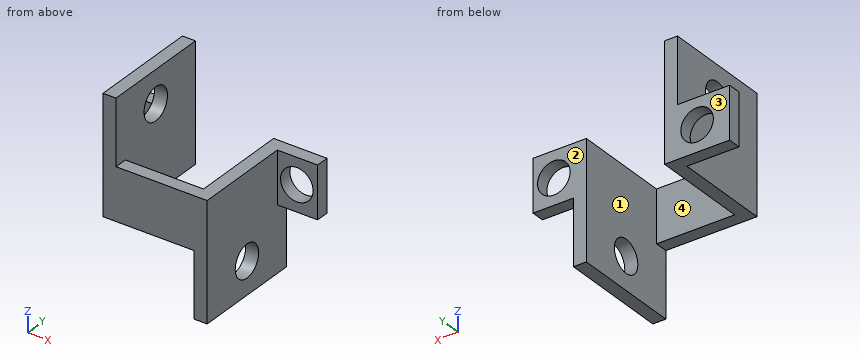
from build123d import *

# Parameters (mm, degrees)
CROQUIS1_W              = 8
CROQUIS1_H              = 2
SALIENTE_EXTRUIR1_DEPTH = 8
CROQUIS2_R              = 2.5
CORTAR_EXTRUIR1_DEPTH   = 2
SKETCH1_W               = 8
SKETCH1_H               = 2
CUT_EXTRUDE1_DEPTH      = 1.8
SKETCH5_W               = 10
SKETCH5_H               = 17
BOSS_EXTRUDE3_DEPTH     = 2
SKETCH6_W               = 10
SKETCH6_H               = 17
SKETCH6_R               = 2.5
BOSS_EXTRUDE4_DEPTH     = 2
SKETCH7_R               = 2.5
CUT_EXTRUDE2_DEPTH      = 2


with BuildPart() as part:
    # Croquis1 → Saliente-Extruir1 (new body)
    with BuildSketch(Plane.XY):
        with Locations((-12, 6.5)):
            Rectangle(CROQUIS1_W, CROQUIS1_H)
        Polygon((-6, 7.5), (-8, 7.5), (-8, 5.5), (-8, -9.5), (8, -9.5), (8, 5.5), (8, 7.5), (6, 7.5), (6, -7.5), (-6, -7.5), align=None)
        with Locations((12, 6.5)):
            Rectangle(CROQUIS1_W, CROQUIS1_H)
    extrude(amount=SALIENTE_EXTRUIR1_DEPTH)

    # Croquis2 → Cortar-Extruir1 (cut)
    with BuildSketch(Plane(origin=(0, 7.5, 0), x_dir=(1, 0, 0), z_dir=(0, 1, 0))):
        with Locations((-11, -4)):
            Circle(CROQUIS2_R)
        with Locations((11, -4)):
            Circle(CROQUIS2_R)
    extrude(amount=-CORTAR_EXTRUIR1_DEPTH, mode=Mode.SUBTRACT)

    # Sketch1 → Cut-Extrude1 (cut)
    with BuildSketch(Plane(origin=(16, 0, 0), x_dir=(0, 0, -1), z_dir=(1, 0, 0))):
        with Locations((-4, 6.5)):
            Rectangle(SKETCH1_W, SKETCH1_H)
    extrude(amount=-CUT_EXTRUDE1_DEPTH, mode=Mode.SUBTRACT)

    # Sketch5 → Boss-Extrude3 (add)
    with BuildSketch(Plane.ZY.offset(8)):
        with Locations((13, -1)):
            Rectangle(SKETCH5_W, SKETCH5_H)
    extrude(amount=-BOSS_EXTRUDE3_DEPTH)

    # Sketch6 → Boss-Extrude4 (add)
    with BuildSketch(Plane(origin=(8, 0, 0), x_dir=(0, 0, -1), z_dir=(1, 0, 0))):
        with Locations((5, -1)):
            Rectangle(SKETCH6_W, SKETCH6_H)
        with Locations((5, -1)):
            Circle(SKETCH6_R, mode=Mode.SUBTRACT)
    extrude(amount=-BOSS_EXTRUDE4_DEPTH)

    # Sketch7 → Cut-Extrude2 (cut)
    with BuildSketch(Plane.ZY.offset(8)):
        with Locations((13, -1)):
            Circle(SKETCH7_R)
    extrude(amount=-CUT_EXTRUDE2_DEPTH, mode=Mode.SUBTRACT)


solid = part.part
Verification items for the finished model (mm, model axes). Face numbers are marked on the shaded views. A direction names the side the tool comes from. Coordinates: 2 decimals unless noted, no trailing zeros. Order: outer loops, then holes, each group sorted by start corner. A loop starts at its lowest first (then second) coordinate and runs counter-clockwise, first axis right, second up. Notation, with made-up numbers: M 68,58.25 L 95,58.25 A17 cw 95,63.25 Z; hole C 57.5,-3.5 d3. An arc over 180 degrees is marked long. Return JSON: item names as keys, results as strings.
1) Cross-section at B-B, the plane x = -11. Record the boundary of the cut face in (y, z), and give its area (3 significant figures).
Answer list:
{"outline": "M 5.5,0 L 7.5,0 L 7.5,1.5 L 5.5,1.5 Z; M 5.5,6.5 L 7.5,6.5 L 7.5,8 L 5.5,8 Z", "area": "6.00 mm2"}
2) Cross-section at A-A, the plane z = 4. Record the boundary of the cut face in (x, y).
Answer list:
{"outline": "M -16,5.5 L -13.5,5.5 L -13.5,7.5 L -16,7.5 Z; M -8.5,5.5 L -8,5.5 L -8,-9.5 L 8,-9.5 L 8,5.5 L 8.5,5.5 L 8.5,7.5 L 6,7.5 L 6,-7.5 L -6,-7.5 L -6,7.5 L -8.5,7.5 Z; M 13.5,5.5 L 14.2,5.5 L 14.2,7.5 L 13.5,7.5 Z"}
3) Access from +Z, -Z, +X, -X, +Y, -Y to the whole of each face (thin tool, end or side, straight path). Record for the marked faces 3 and 4.
Answer list:
{"face 3": "+Z, -Z, +X, -X, +Y", "face 4": "+Z, -Z, +Y"}
4) Cross-section at D-D, the plane z = -5. Record the boundary of the cut face in (x, y), and give its area (3 significant figures).
Answer list:
{"outline": "M 6,-9.5 L 8,-9.5 L 8,-3.5 L 6,-3.5 Z; M 6,1.5 L 8,1.5 L 8,7.5 L 6,7.5 Z", "area": "24.0 mm2"}
5) Release check for a two-part mould opening along X. For the marked faces 1 and 2 record: +X half, -X half, draft (parallel to the pull), parting line (faces both ways), or undercut.
Answer list:
{"face 1": "undercut", "face 2": "draft"}
6) Gauge pin test, flat ends, axial feed: pin 1 (2 mm diameter, centred on y = -7, z = -6, fed in from +X); pin 2 (5 mm diameter, centred on x = 11.5, z = 5.5, fed in from -Y); pin 3 (8.5 mm diameter, centred on y = -0.5, z = 0.5, fed in from -X). Record the tip position at first contact, or that the pin passes through.
Answer list:
{"pin 1": "x = 8", "pin 2": "y = 5.5", "pin 3": "x = -8"}
7) Thickness scan on L1, parallel to X at y = 6.6, z = 4; L2, parallel to X at y = -2.5, z = 6; L3, parallel to Z at x = 11, y = 6.7. Record the ranges inside material, lowest first. Write a range as [from, to].
Answer list:
{"L1": "[-16, -13.5], [-8.5, -6], [6, 8.5], [13.5, 14.2]", "L2": "[-8, -6], [6, 8]", "L3": "[0, 1.5], [6.5, 8]"}
8) Cross-section at C-C, the plane y = -1. Record the boundary of the cut face in (x, z), and give its area (3 significant figures).
Answer list:
{"outline": "M -8,0 L -6,0 L -6,10.5 L -8,10.5 Z; M -8,15.5 L -6,15.5 L -6,18 L -8,18 Z; M 6,-10 L 8,-10 L 8,-7.5 L 6,-7.5 Z; M 6,-2.5 L 8,-2.5 L 8,8 L 6,8 Z", "area": "52.0 mm2"}
